Can you work these out from the model? Positions are in its coordinate system, mm. Face numbers are marked on the shaded views. A direction names the side the tool comes from. Give positions to 0.01 mm unless a question says otherwise; leave off trailing zeros. Loops run counter-clockwise (first coordinate to the right, second up) from the corner with the lowest first, then second, coordinate; pieces in that order, holes last. Notation, with made-up numbers: M 38.5,7.25 L 78.5,7.25 A25 cw 78.5,36.25 Z; hole C 89.5,59.5 d5. An arc over 180 degrees is marked long. Use CSV: the item, a comma, the result in double quotes.
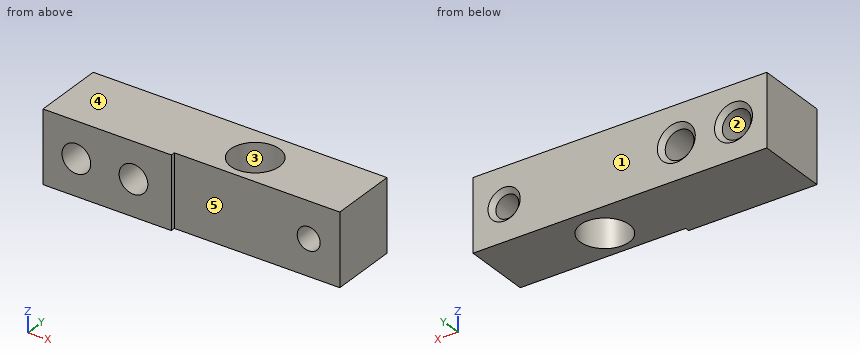
from build123d import *

# Parameters (mm, degrees)
SKETCH1_W           = 31.9024
SKETCH1_H           = 31.6992
BOSS_EXTRUDE1_DEPTH = 129.921
SKETCH2_W           = 73.1774
SKETCH2_H           = 31.9024
CUT_EXTRUDE1_DEPTH  = 1.8796
SKETCH4_R           = 6.35
SKETCH4_R_2         = 5.08
CUT_EXTRUDE2_DEPTH  = 135.68016299
CHAMFER2_SIZE       = 2.032
SKETCH9_R           = 10.836935607
CUT_EXTRUDE3_DEPTH  = 135.716143008


with BuildPart() as part:
    # Sketch1 → Boss-Extrude1 (new body)
    with BuildSketch(Plane(origin=(0, 0, 0), x_dir=(0, 0, -1), z_dir=(1, 0, 0))):
        Rectangle(SKETCH1_W, SKETCH1_H)
    extrude(amount=BOSS_EXTRUDE1_DEPTH)

    # Sketch2 → Cut-Extrude1 (cut)
    with BuildSketch(Plane.XZ.offset(15.8496)):
        with Locations((93.3323, 0)):
            Rectangle(SKETCH2_W, SKETCH2_H)
    extrude(amount=-CUT_EXTRUDE1_DEPTH, mode=Mode.SUBTRACT)

    # Sketch4 → Cut-Extrude2 (cut, through all)
    with BuildSketch(Plane(origin=(0, 15.8496, 0), x_dir=(1, 0, 0), z_dir=(0, 1, 0))):
        with Locations(Location((40.005, 0, 0), (0, 0, 270))):
            Circle(SKETCH4_R)
        with Locations(Location((14.732, 0, 0), (0, 0, 270))):
            Circle(SKETCH4_R)
        with Locations(Location((116.1669, 0, 0), (0, 0, 270))):
            Circle(SKETCH4_R_2)
    extrude(amount=-CUT_EXTRUDE2_DEPTH, mode=Mode.SUBTRACT)

    # Chamfer2
    chamfer2_edges = [part.edges().sort_by_distance(p)[0] for p in [
        (116.1669, 15.8496, -5.08),
        (14.732, 15.8496, -6.35),
        (40.005, 15.8496, -6.35),
    ]]
    chamfer(chamfer2_edges, length=CHAMFER2_SIZE)

    # Sketch9 → Cut-Extrude3 (cut, through all)
    with BuildSketch(Plane(origin=(0, 0, -15.9512), x_dir=(-1, 0, 0), z_dir=(0, 0, -1))):
        with Locations((-82.727824096, 0)):
            Circle(SKETCH9_R)
    extrude(amount=-CUT_EXTRUDE3_DEPTH, mode=Mode.SUBTRACT)


solid = part.part
Q1. For the marked faces 4 and 5, which set-ups out of +Z, -Z, +X, -X, +Y, -Y let a thin tool reach every point of the face, with its end or its side?
Model answer:
face 4,"+Z, +X, -X, +Y, -Y"
face 5,"+Z, -Z, +X, -Y"
Q2. I want a section at C-C, the plane z = -12.5. Please give me the cut outline in (x, y).
Model answer:
outline,"M 0,-15.85 L 56.74,-15.85 L 56.74,-13.97 L 129.92,-13.97 L 129.92,15.85 L 0,15.85 Z; hole C 82.73,0 d21.67"
Q3. I want a section at D-D, the plane y = -12.5. Please give me the cut outline in (x, z) (3 decimals).
Model answer:
outline,"M 0,-15.951 L 129.921,-15.951 L 129.921,15.951 L 0,15.951 Z; hole C 14.732,0 d12.7; hole C 40.005,0 d12.7; hole C 116.167,0 d10.16"
Q4. I want a section at B-B, the plane y = 0. Please give me the cut outline in (x, z) (3 decimals), then the cut area to 3 significant figures.
Model answer:
outline,"M 0,-15.951 L 71.891,-15.951 L 71.891,15.951 L 0,15.951 Z; M 93.565,-15.951 L 129.921,-15.951 L 129.921,15.951 L 93.565,15.951 Z; hole C 14.732,0 d12.7; hole C 40.005,0 d12.7; hole C 116.167,0 d10.16"
area,"3,120 mm2"
Q5. I'm going to push flat-ended pins straight in: P1, Ø6, axis at y = -12, z = -4.5, coming from the -X side; P2, Ø1.5, axis at y = -15, z = 5, coming from the +X side; P3, Ø16.5, axis at x = 116.17, z = 0, coming from the -Y side. Where does each tip first touch, or does it pass through?
Model answer:
P1,"x = 0"
P2,"x = 56.74"
P3,"y = -13.97"
Q6. If we mould it in two halves opening along Y, with no side actions, what happens to the marked faces 1, 2 and 3? For each: released by +Y, released by -Y, zero draft, split by the parting line, or undercut.
Model answer:
face 1,"released by +Y"
face 2,"zero draft"
face 3,"undercut"
Q7. Please list where these lines run through material, in increasing order: L1, parallel to X at y = -12, z = -4; L2, parallel to X at y = -6, z = 0 (3 decimals); L3, parallel to Y at x = 71.5, z = 6. Write a range as from..to.
Model answer:
L1,"0..9.8, 19.66..35.07, 44.94..113.04, 119.3..129.92"
L2,"0..8.382, 21.082..33.655, 46.355..73.703, 91.752..111.087, 121.247..129.921"
L3,"-13.97..15.85"
Q8. I want a section at A-A, the plane z = 0. Please give me the cut outline in (x, y) (3 decimals), then the cut area to 3 significant figures.
Model answer:
outline,"M 0,-15.85 L 8.382,-15.85 L 8.382,13.818 L 6.35,15.85 L 0,15.85 Z; M 21.082,-15.85 L 33.655,-15.85 L 33.655,13.818 L 31.623,15.85 L 23.114,15.85 L 21.082,13.818 Z; M 46.355,-15.85 L 56.744,-15.85 L 56.744,-13.97 L 111.087,-13.97 L 111.087,13.818 L 109.055,15.85 L 48.387,15.85 L 46.355,13.818 Z; M 121.247,-13.97 L 129.921,-13.97 L 129.921,15.85 L 123.279,15.85 L 121.247,13.818 Z; hole C 82.728,0 d21.674"
area,"2,490 mm2"
